from build123d import *

# Parameters (mm, degrees)
F0_W     = 100
F0_H     = 100
F1_DEPTH = 50
F2_W     = 60
F2_H     = 60
F3_DEPTH = 30
F4_W     = 30
F4_H     = 30
F5_DEPTH = 30
F6_SIZE  = 2


with BuildPart() as f1:
    # F0 (on Top) → F1 (new body)
    with BuildSketch(Plane.XY):
        Rectangle(F0_W, F0_H)
    extrude(amount=F1_DEPTH)

    # F2 (on face) → F3 (cut)
    with BuildSketch(Plane.XY.offset(50)):
        Rectangle(F2_W, F2_H)
    extrude(amount=-F3_DEPTH, mode=Mode.SUBTRACT)

    # F4 (on face) → F5 (cut)
    with BuildSketch(Plane.XY.offset(50)):
        with Locations((-35, 35)):
            Rectangle(F4_W, F4_H)
        with Locations((-35, -35)):
            Rectangle(F4_W, F4_H)
        with Locations((35, -35)):
            Rectangle(F4_W, F4_H)
        with Locations((35, 35)):
            Rectangle(F4_W, F4_H)
    extrude(amount=-F5_DEPTH, mode=Mode.SUBTRACT)

    # F6
    f6_edges = [f1.edges().sort_by_distance(p)[0] for p in [
        (0, -50, 50),
        (50, 0, 50),
        (0, 50, 50),
        (-50, 0, 50),
    ]]
    chamfer(f6_edges, length=F6_SIZE)


solid = f1.part
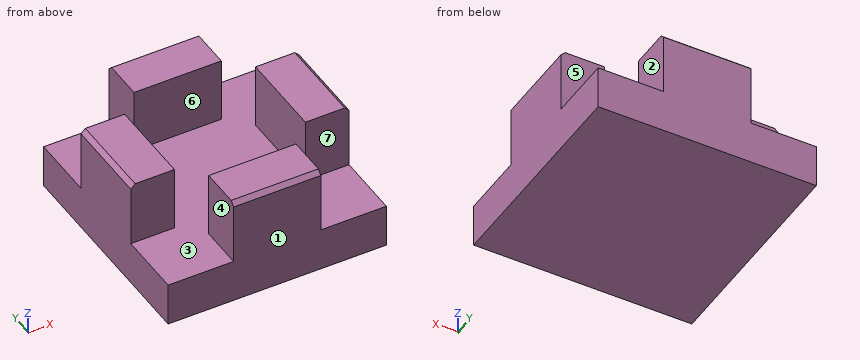
Verification items for the finished model (mm, model axes). Face numbers are marked on the shaded views. A direction names the side the tool comes from. Round coordinates to 2 decimals unless told otherwise and drop trailing zeros. Loops run counter-clockwise (first coordinate to the right, second up) from the corner with the lowest first, then second, coordinate; pieces in that order, holes last. Notation, with made-up numbers: (-2, 62.5) - (18, 62.5) arc R17 ccw to (18, 77.5) - close; hole circle Ø2 at (43, 56). An arc over 180 degrees is marked (long way). Answer in a Markdown table with one row per item. Add a question column.
Q1. Material ranges on line 1 (Y direction, x = -9, z = 47.5); line 2 (X direction, y = 43, z = 40.5), recorded low to high.
Q2. Tool access check on the marked faces 4, 5, 6 and 7. Record the directions out of +Z, -Z, +X, -X, +Y, -Y that give a thin tool (end or side, any length) a straight path to the whole face; none if there is none.
Q3. Release check for a two-part mould opening along Y. For the marked faces 1, 2 and 3 record: pulls with the +Y half, pulls with the -Y half, needs draft (parallel to the pull), parting line crosses it, or undercut.
Q4. Section check A-A on z = 46.5. Enter the section's corners in (x, y).
Q5. Section check D-D on y = -36.5. Enter the section's corners in (x, z).
Q6. Section check B-B on y = 2. Enter the section's corners in (x, z).
Q7. Gauge pin test, flat ends, axial feed: pin 1 (6 mm diameter, centred on x = -39, z = 28.5, fed in from +Y); pin 2 (4 mm diameter, centred on y = -38.5, z = 27, fed in from +X); pin 3 (10 mm diameter, centred on x = -45, z = 36, fed in from -Y). Record the tip position at first contact, or that the pin passes through.
Found:
| question | item | result |
|---|---|---|
| 1 | line 1 | y = -50 to -30, 30 to 50 |
| 1 | line 2 | x = -20 to 20 |
| 2 | face 4 | +Z, -X, +Y, -Y |
| 2 | face 5 | +Z, +X, -X, +Y |
| 2 | face 6 | +Z, +X, -X |
| 2 | face 7 | +Z, +X, -X, -Y |
| 3 | face 1 | pulls with the -Y half |
| 3 | face 2 | needs draft |
| 3 | face 3 | undercut |
| 4 | outline | (-50, -20) - (-30, -20) - (-30, 20) - (-50, 20) - close; (-20, -50) - (20, -50) - (20, -30) - (-20, -30) - close; (-20, 30) - (20, 30) - (20, 50) - (-20, 50) - close; (30, -20) - (50, -20) - (50, 20) - (30, 20) - close |
| 5 | outline | (-50, 0) - (50, 0) - (50, 20) - (20, 20) - (20, 50) - (-20, 50) - (-20, 20) - (-50, 20) - close |
| 6 | outline | (-50, 0) - (50, 0) - (50, 48) - (48, 50) - (30, 50) - (30, 20) - (-30, 20) - (-30, 50) - (-48, 50) - (-50, 48) - close |
| 7 | pin 1 | stops at y = 20 |
| 7 | pin 2 | stops at x = 20 |
| 7 | pin 3 | stops at y = -20 |
